Work out the finished part from the listing and answer in its coordinate system (mm). Face numbers are marked on the shaded views. A direction names the side the tool comes from. Give positions to 0.01 mm unless a question says otherwise; leave off trailing zeros. Order: outer loops, then holes, each group sorted by start corner. A loop starts at its lowest first (then second) coordinate and runs counter-clockwise, first axis right, second up.
```python
from build123d import *

# Parameters (mm, degrees)
BOSS_EXTRUDE1_DEPTH                        = 4
BOSS_EXTRUDE1_DEPTH_BACK                   = 3
SKETCH1_R                                  = 34
SKETCH1_R_2                                = 1
SKETCH1_R_3                                = 7
CUT_EXTRUDE1_REACH                         = 50.59
CUT_EXTRUDE2_REACH                         = 50.744
FILLET1_R                                  = 5
FILLET2_R                                  = 4
M2_5X0_45_TAPPED_HOLE1_D                   = 2.05
CBORE_FOR_M2_5_PAN_HEAD_SCREW1_D           = 2.9
CBORE_FOR_M2_5_PAN_HEAD_SCREW1_DEPTH       = 7
CBORE_FOR_M2_5_PAN_HEAD_SCREW1_CBORE_D     = 6
CBORE_FOR_M2_5_PAN_HEAD_SCREW1_CBORE_DEPTH = 2.1
SKETCH13_R                                 = 2.2
CUT_EXTRUDE3_DEPTH                         = 3
CUT_EXTRUDE4_REACH                         = 50.59
FILLET3_R                                  = 2
CUT_EXTRUDE5_DEPTH                         = 3
FILLET4_R                                  = 2
CUT_EXTRUDE7_DEPTH                         = 2
FILLET5_R                                  = 2


with BuildPart() as part:
    # Sketch1 → Boss-Extrude1 (new, two sides: drawn at the far end of the back side and taken through both)
    with BuildSketch(Plane.XY.offset(-BOSS_EXTRUDE1_DEPTH_BACK)):
        Circle(SKETCH1_R)
        with Locations((-27.5, 0)):
            Circle(SKETCH1_R_2, mode=Mode.SUBTRACT)
        with Locations((13.75, 23.815698604)):
            Circle(SKETCH1_R_2, mode=Mode.SUBTRACT)
        with Locations((13.75, -23.815698604)):
            Circle(SKETCH1_R_2, mode=Mode.SUBTRACT)
        Circle(SKETCH1_R_3, mode=Mode.SUBTRACT)
    extrude(amount=BOSS_EXTRUDE1_DEPTH + BOSS_EXTRUDE1_DEPTH_BACK)

    # Sketch2 → Cut-Extrude1 (cut, up to next)
    with BuildSketch(Plane.XY.offset(4), mode=Mode.PRIVATE) as cut_extrude1_sk1:
        with BuildLine():
            Line((33.466401061, 6), (25, 6))
            Line((25, 6), (25, -6))
            Line((25, -6), (33.466401061, -6))
            ThreePointArc((33.466401061, -6), (34, 0), (33.466401061, 6))
        make_face()
    cut_extrude1_tool1 = extrude(cut_extrude1_sk1.sketch, amount=-CUT_EXTRUDE1_REACH, mode=Mode.PRIVATE) & part.part
    add(cut_extrude1_tool1.solids().sort_by_distance((29.412779, 0, 4))[0], mode=Mode.SUBTRACT)

    # Sketch4 → Cut-Extrude2 (cut, up to next)
    with BuildSketch(Plane.XY.offset(-4), mode=Mode.PRIVATE) as cut_extrude2_sk1:
        with BuildLine():
            Line((-24.229587732, -23.852192317), (-22.452552523, -18.173755396))
            Line((-22.452552523, -18.173755396), (8.086940161, -27.730919545))
            Line((8.086940161, -27.730919545), (6.309904952, -33.409356466))
            ThreePointArc((6.309904952, -33.409356466), (-10.154486908, -32.448210977), (-24.229587732, -23.852192317))
        make_face()
    cut_extrude2_tool1 = extrude(cut_extrude2_sk1.sketch, amount=CUT_EXTRUDE2_REACH, mode=Mode.PRIVATE) & part.part
    add(cut_extrude2_tool1.solids().sort_by_distance((-8.498569, -27.1568, -4))[0], mode=Mode.SUBTRACT)

    # Fillet1
    fillet1_edges = [part.edges().sort_by_distance(p)[0] for p in [
        (33.466401061, 6, 0.5),
        (33.466401061, -6, 0.5),
    ]]
    fillet(fillet1_edges, radius=FILLET1_R)

    # Fillet2
    fillet2_edges = [part.edges().sort_by_distance(p)[0] for p in [
        (25, -6, 0.5),
        (25, 6, 0.5),
    ]]
    fillet(fillet2_edges, radius=FILLET2_R)

    # M2.5x0.45 Tapped Hole1 (through all)
    with Locations(Plane.XY.offset(4)):
        with Locations((-25.95639466, -15.977032774), (12.217971196, -27.92348796), (23.567103623, 8.342159603), (-14.607262233, 20.288614789)):
            Hole(M2_5X0_45_TAPPED_HOLE1_D / 2)

    # CBORE for M2.5 Pan Head Screw1
    with Locations(Plane.XY.offset(4)):
        with Locations((-27.5, 0), (13.75, 23.815698604), (13.75, -23.815698604)):
            CounterBoreHole(CBORE_FOR_M2_5_PAN_HEAD_SCREW1_D / 2, CBORE_FOR_M2_5_PAN_HEAD_SCREW1_CBORE_D / 2, CBORE_FOR_M2_5_PAN_HEAD_SCREW1_CBORE_DEPTH, depth=CBORE_FOR_M2_5_PAN_HEAD_SCREW1_DEPTH)

    # Sketch13 → Cut-Extrude3 (cut)
    with BuildSketch(Plane(origin=(0, 0, -3), x_dir=(-1, 0, 0), z_dir=(0, 0, -1))):
        with Locations((-13.75, 23.815698604)):
            Circle(SKETCH13_R)
        with Locations((27.5, 0)):
            Circle(SKETCH13_R)
        with Locations((-13.75, -23.815698604)):
            Circle(SKETCH13_R)
    extrude(amount=-CUT_EXTRUDE3_DEPTH, mode=Mode.SUBTRACT)

    # Sketch14 → Cut-Extrude4 (cut, up to next)
    with BuildSketch(Plane.XY.offset(4), mode=Mode.PRIVATE) as cut_extrude4_sk1:
        with BuildLine():
            Line((-5.976383774, 33.47062648), (-12.295486181, 13.278215978))
            Line((-12.295486181, 13.278215978), (1.065541868, 9.096956663))
            Line((1.065541868, 9.096956663), (8.519375308, 32.915349677))
            ThreePointArc((8.519375308, 32.915349677), (1.301454789, 33.975082273), (-5.976383774, 33.47062648))
        make_face()
    cut_extrude4_tool1 = extrude(cut_extrude4_sk1.sketch, amount=-CUT_EXTRUDE4_REACH, mode=Mode.PRIVATE) & part.part
    add(cut_extrude4_tool1.solids().sort_by_distance((-1.905533, 22.418355, 4))[0], mode=Mode.SUBTRACT)

    # Fillet3
    fillet3_edges = [part.edges().sort_by_distance(p)[0] for p in [
        (-5.976383774, 33.47062648, 0.5),
        (8.519375308, 32.915349677, 0.5),
        (1.065541868, 9.096956663, 0.5),
        (-12.295486181, 13.278215978, 0.5),
        (-24.229587732, -23.852192317, 0.5),
        (6.309904952, -33.409356466, 0.5),
        (8.086940161, -27.730919545, 0.5),
        (-22.452552523, -18.173755396, 0.5),
    ]]
    fillet(fillet3_edges, radius=FILLET3_R)

    # Sketch15 → Cut-Extrude5 (cut)
    with BuildSketch(Plane.XY.offset(4)):
        Polygon((6.448401058, -32.966798325), (10.028239129, -21.527585094), (-20.511253555, -11.970420945), (-24.091091627, -23.409634176), align=None)
    extrude(amount=-CUT_EXTRUDE5_DEPTH, mode=Mode.SUBTRACT)

    # Fillet4
    fillet4_edges = [part.edges().sort_by_distance(p)[0] for p in [
        (10.028239129, -21.527585094, 2.5),
        (-20.511253555, -11.970420945, 2.5),
    ]]
    fillet(fillet4_edges, radius=FILLET4_R)

    # Sketch16 → Cut-Extrude7 (cut)
    with BuildSketch(Plane.XY.offset(4)):
        with BuildLine():
            Line((20.035974781, 9.447206707), (2.857510146, 14.823111541))
            Line((2.857510146, 14.823111541), (4.052155665, 18.640548127))
            Line((4.052155665, 18.640548127), (21.2306203, 13.264643293))
            ThreePointArc((21.2306203, 13.264643293), (22.542015833, 10.758602241), (20.035974781, 9.447206707))
        make_face()
    extrude(amount=-CUT_EXTRUDE7_DEPTH, mode=Mode.SUBTRACT)

    # Fillet5
    fillet5_edges = [part.edges().sort_by_distance(p)[0] for p in [
        (2.857510146, 14.823111541, 3),
        (4.052155665, 18.640548127, 3),
    ]]
    fillet(fillet5_edges, radius=FILLET5_R)


solid = part.part
```
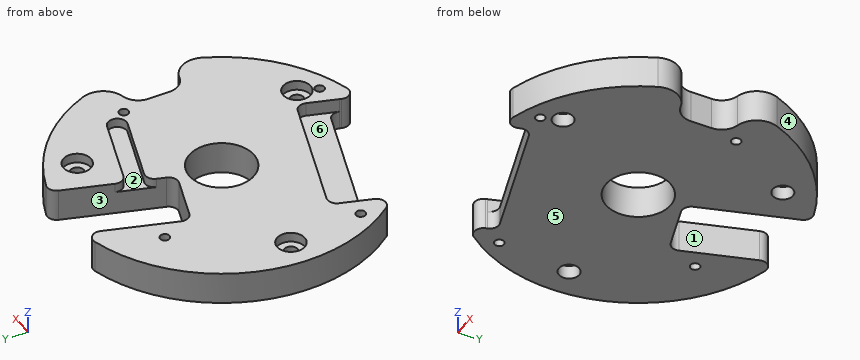
1. The mould has two halves that part along X. Classify the marked faces 4, 5 and 6: pulls with the +X half, pulls with the -X half, needs draft (parallel to the pull), parting line crosses it, or undercut.
Findings below:
face 4: pulls with the +X half
face 5: needs draft
face 6: undercut
2. Straight lines are drawn through the part: probe 1 along X at (y, z) = (25, 2.5); probe 2 along Y at (x, z) = (13.75, 3.3); probe 3 along X at (y, z) = (9, 1.25). For each, find the intervals that lie inside material, in ascending order.
Findings below:
probe 1: x = -23.04 to -8.63, 6.04 to 10.99, 16.51 to 23.04
probe 2: y = -31.1 to -26.82, -20.82 to 11.41, 15.61 to 20.82, 26.82 to 31.1
probe 3: x = -32.79 to 22.78, 24.35 to 31.42
3. Which of the six approach directions +Z, -Z, +X, -X, +Y, -Y give full straight-line access (tool end or side, diameter ignored) to the marked faces 1, 2 and 3?
Findings below:
face 1: +Z, -Z
face 2: +Z
face 3: +Z, -Z, +Y
4. The part is cut by section C-C (z = -1.25). State how many separate pieces and enclosed holes the cut face has, then the cut area to 3 significant figures.
Findings below:
separate pieces: 1
enclosed holes: 8
area: 2,680 mm2
5. The part is cut by section A-A (y = 0). Write down the section's boundary in (x, z).
Findings below:
outline: (-34, -3) - (-29.7, -3) - (-29.7, 0) - (-28.95, 0) - (-28.95, 1.9) - (-30.5, 1.9) - (-30.5, 4) - (-34, 4) - close; (-26.05, 0) - (-25.3, 0) - (-25.3, -3) - (-7, -3) - (-7, 4) - (-24.5, 4) - (-24.5, 1.9) - (-26.05, 1.9) - close; (7, -3) - (25, -3) - (25, 4) - (7, 4) - close
6. The part is cut by section D-D (y = -8). Write down the section's boundary in (x, z), then the cut area to 3 significant figures.
Findings below:
outline: (-33.05, -3) - (30.83, -3) - (30.83, 4) - (-33.05, 4) - close
area: 447 mm2
7. Given P1, Ø3.5, axis at x = 13.75, y = -23.82, coming from the -Z side; P2, Ø1, axis at x = -1.5, z = 1.5, coming from the +Y side; P3, Ø12.5, axis at x = 15.5, y = 15, coming from the +Z side; P4, Ø1.5, axis at x = 4.5, y = -23, coming from the +Z side, each flat-ended and moving along its own axis, determine where each tip first touches the part or whether it passes through.
Findings below:
P1: stops at z = 0
P2: stops at y = 10.06
P3: stops at z = 4
P4: stops at z = 1
8. The part is cut by section B-B (x = 0). Write down the section's boundary in (y, z).
Findings below:
outline: (-25.2, -3) - (-7, -3) - (-7, 4) - (-18.39, 4) - (-18.39, 1) - (-25.2, 1) - close; (7, -3) - (9.62, -3) - (9.62, 4) - (7, 4) - close
